Source: CAD feature listing. Evaluate the final solid. Frame: model axes, mm. Face numbers are marked on the shaded views. A direction names the side the tool comes from. Give positions to 0.01 mm unless a question says otherwise; leave off trailing zeros. Loops run counter-clockwise (first coordinate to the right, second up) from the corner with the lowest first, then second, coordinate; pieces in that order, holes last. Notation, with made-up numbers: M 17.5,12.5 L 55.5,12.5 A22 cw 55.5,25.5 Z; hole C 30.25,60.5 d5. An arc over 180 degrees is marked long. Write item = value, one per line.
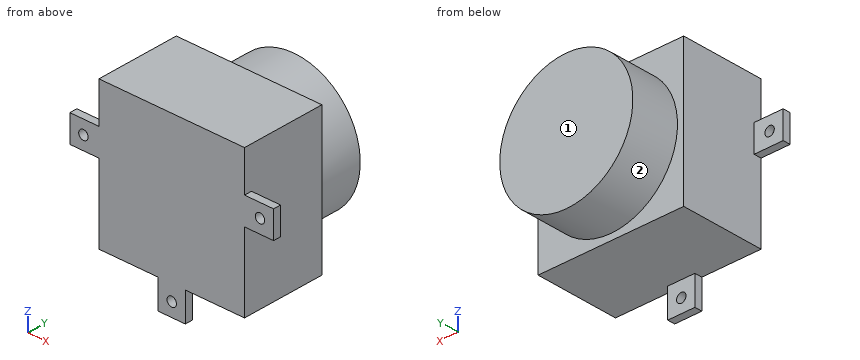
from build123d import *

# Parameters (mm, degrees)
SK_HOUSING_W       = 38.59
SK_HOUSING_H       = 38.59
EX_HOUSING_DEPTH   = 22.2
SK_EARS_W          = 8
SK_EARS_H          = 7.2
SK_EARS_W_2        = 7.2
SK_EARS_H_2        = 8
EX_EARS_DEPTH      = 2
SK_HOLES_3X_R      = 1.25
CUT_HOLES_3X_DEPTH = 2
SK_DOME_R          = 17.645
EX_DOME_DEPTH      = 12.8


with BuildPart() as part:
    # SK_Housing → EX_Housing (new body)
    with BuildSketch(Plane(origin=(0, 0, 0), x_dir=(1, 0, 0), z_dir=(0, 1, 0))):
        Rectangle(SK_HOUSING_W, SK_HOUSING_H)
    extrude(amount=EX_HOUSING_DEPTH)

    # SK_Ears → EX_Ears (add)
    with BuildSketch(Plane(origin=(0, 0, 0), x_dir=(1, 0, 0), z_dir=(0, 1, 0))):
        with Locations((23, -4.93)):
            Rectangle(SK_EARS_W, SK_EARS_H)
        with Locations((-23, -4.93)):
            Rectangle(SK_EARS_W, SK_EARS_H)
        with Locations((0, 23)):
            Rectangle(SK_EARS_W_2, SK_EARS_H_2)
    extrude(amount=EX_EARS_DEPTH)

    # SK_Holes_3x → CUT_Holes_3x (cut)
    with BuildSketch(Plane(origin=(0, 0, 0), x_dir=(1, 0, 0), z_dir=(0, 1, 0))):
        with Locations(Location((23.4, -4.93, 0), (0, 0, 270))):
            Circle(SK_HOLES_3X_R)
        with Locations(Location((-23.4, -4.93, 0), (0, 0, 270))):
            Circle(SK_HOLES_3X_R)
        with Locations(Location((0, 23.39, 0), (0, 0, 270))):
            Circle(SK_HOLES_3X_R)
    extrude(amount=CUT_HOLES_3X_DEPTH, mode=Mode.SUBTRACT)

    # SK_Dome → EX_Dome (add)
    with BuildSketch(Plane(origin=(0, 22.2, 0), x_dir=(1, 0, 0), z_dir=(0, 1, 0))):
        with Locations(Location((0, 0, 0), (0, 0, 270))):
            Circle(SK_DOME_R)
    extrude(amount=EX_DOME_DEPTH)


solid = part.part
1. Cut plane A-A, the plane x = 0. Return the cut outline in (y, z) (3 decimals), then the cut area to 3 significant figures.
Derived:
outline = M 0,-27 L 2,-27 L 2,-24.64 L 0,-24.64 Z; M 0,-22.14 L 2,-22.14 L 2,-19.295 L 22.2,-19.295 L 22.2,-17.645 L 35,-17.645 L 35,17.645 L 22.2,17.645 L 22.2,19.295 L 0,19.295 Z
area = 1,320 mm²
2. Cut plane C-C, the plane z = 0. Return the cut outline in (x, y) (3 decimals), then the cut area to 3 significant figures.
Derived:
outline = M -19.295,0 L 19.295,0 L 19.295,22.2 L 17.645,22.2 L 17.645,35 L -17.645,35 L -17.645,22.2 L -19.295,22.2 Z
area = 1,310 mm²
3. Material intervals for probe 1 along X at (y, z) = (1.1, 4.93); probe 2 along X at (y, z) = (3, -9.5) (3 decimals), sorted ascending. Write a range as from..to.
Derived:
probe_1 = -27..-24.65, -22.15..22.15, 24.65..27
probe_2 = -19.295..19.295
4. Cut plane B-B, the plane z = -23.39. Return the cut outline in (x, y).
Derived:
outline = M -3.6,0 L -1.25,0 L -1.25,2 L -3.6,2 Z; M 1.25,0 L 3.6,0 L 3.6,2 L 1.25,2 Z
5. Cut plane D-D, the plane x = 23.4. Return the cut outline in (y, z), then the cut area to 3 significant figures.
Derived:
outline = M 0,1.33 L 2,1.33 L 2,3.68 L 0,3.68 Z; M 0,6.18 L 2,6.18 L 2,8.53 L 0,8.53 Z
area = 9.40 mm²
6. Reachability of the marked faces 1 and 2 from +Z, -Z, +X, -X, +Y, -Y: full face, straight path, thin tool, end or side. Return the list, or none.
Derived:
face_1 = +Z, -Z, +X, -X, +Y
face_2 = +Y
7. First-contact query: pin 1 Ø1.6 at (x, y) = (-21.5, 0.5) entering from -Z; pin 2 Ø1 at (y, z) = (1, -23.5) entering from -X; pin 3 Ø3.5 at (x, z) = (24.5, 5) entering from +Y. Flat tips, straight axial feed; report the tip coordinate or a pass-through.
Derived:
pin_1 = 1.33
pin_2 = -3.6
pin_3 = 2
